```python
from build123d import *

# Parameters (mm, degrees)
SKETCH1_R           = 4
SKETCH1_R_2         = 1.5
SKETCH1_R_3         = 2.5
BOSS_EXTRUDE1_DEPTH = 4


with BuildPart() as part:
    # Sketch1 → Boss-Extrude1 (new body)
    with BuildSketch(Plane.XY):
        with BuildLine():
            Line((12.000000461, 24.00000011), (133.000000461, 24.00000011))
            ThreePointArc((133.000000461, 24.00000011), (145.000000461, 12.00000011), (133.000000461, 1.1e-07))
            Line((133.000000461, 1.1e-07), (12.000000461, 1.1e-07))
            ThreePointArc((12.000000461, 1.1e-07), (4.61e-07, 12.00000011), (12.000000461, 24.00000011))
        make_face()
        with Locations((12.000000461, 12.00000011)):
            Circle(SKETCH1_R, mode=Mode.SUBTRACT)
        with Locations((60.000000461, 5.00000011)):
            Circle(SKETCH1_R_2, mode=Mode.SUBTRACT)
        with Locations((60.000000461, 19.00000011)):
            Circle(SKETCH1_R_2, mode=Mode.SUBTRACT)
        with Locations((85.000000461, 5.00000011)):
            Circle(SKETCH1_R_2, mode=Mode.SUBTRACT)
        with Locations((85.000000461, 19.00000011)):
            Circle(SKETCH1_R_2, mode=Mode.SUBTRACT)
        with Locations((133.000000461, 12.00000011)):
            Circle(SKETCH1_R_3, mode=Mode.SUBTRACT)
        with BuildLine():
            ThreePointArc((9.729668922, 4.433322836), (12.000000461, 4.100062751), (14.270331999, 4.433322836))
            ThreePointArc((14.270331999, 4.433322836), (14.500023689, 5.017172326), (14.000000461, 5.396138381))
            ThreePointArc((14.000000461, 5.396138381), (12.000000461, 5.09992839), (10.000000461, 5.396138381))
            ThreePointArc((10.000000461, 5.396138381), (9.499977232, 5.017172326), (9.729668922, 4.433322836))
        make_face(mode=Mode.SUBTRACT)
        with BuildLine():
            ThreePointArc((19.566677735, 9.729668571), (19.899937819, 12.00000011), (19.566677735, 14.270331648))
            ThreePointArc((19.566677735, 14.270331648), (18.982828244, 14.500023338), (18.603862189, 14.00000011))
            ThreePointArc((18.603862189, 14.00000011), (18.90007218, 12.00000011), (18.603862189, 10.00000011))
            ThreePointArc((18.603862189, 10.00000011), (18.982828244, 9.499976882), (19.566677735, 9.729668571))
        make_face(mode=Mode.SUBTRACT)
        with BuildLine():
            ThreePointArc((14.270331999, 19.566677384), (12.000000461, 19.899937468), (9.729668922, 19.566677384))
            ThreePointArc((9.729668922, 19.566677384), (9.499977232, 18.982827894), (10.000000461, 18.603861839))
            ThreePointArc((10.000000461, 18.603861839), (12.000000461, 18.900071829), (14.000000461, 18.603861839))
            ThreePointArc((14.000000461, 18.603861839), (14.500023689, 18.982827894), (14.270331999, 19.566677384))
        make_face(mode=Mode.SUBTRACT)
        with BuildLine():
            ThreePointArc((4.433323186, 14.270331648), (4.100063102, 12.00000011), (4.433323186, 9.729668571))
            ThreePointArc((4.433323186, 9.729668571), (5.017172677, 9.499976882), (5.396138732, 10.00000011))
            ThreePointArc((5.396138732, 10.00000011), (5.099928741, 12.00000011), (5.396138732, 14.00000011))
            ThreePointArc((5.396138732, 14.00000011), (5.017172677, 14.500023338), (4.433323186, 14.270331648))
        make_face(mode=Mode.SUBTRACT)
    extrude(amount=BOSS_EXTRUDE1_DEPTH)


solid = part.part
```
For this review, take the finished solid that the model builds, in its own axes (mm). A direction names the side the tool comes from. Coordinates: 2 decimals unless noted, no trailing zeros. Order: outer loops, then holes, each group sorted by start corner. A loop starts at its lowest first (then second) coordinate and runs counter-clockwise, first axis right, second up. Notation, with made-up numbers: (30.25, 17) -> (45.25, 17) arc R21 cw to (45.25, 26) -> close; hole circle Ø1 at (62.5, 37). An arc over 180 degrees is marked (long way). Answer as CSV lines item,"result".
Q1. For faces 1 (the face through (19.9, 12, 2)), 2 (the face through (73, 0, 2)), list the 3-axis set-ups (+Z, -Z, +X, -X, +Y, -Y) from which the entire face can be reached by the end or side of a thin tool; tool diameter is ignored.
Model answer:
face 1,"+Z, -Z"
face 2,"+Z, -Z, +X, -X, -Y"
Q2. We need section A-A (y = 12). State the section outline as (x, z) points, plus the area to 3 significant figures.
Model answer:
outline,"(0, 0) -> (4.1, 0) -> (4.1, 4) -> (0, 4) -> close; (5.1, 0) -> (8, 0) -> (8, 4) -> (5.1, 4) -> close; (16, 0) -> (18.9, 0) -> (18.9, 4) -> (16, 4) -> close; (19.9, 0) -> (130.5, 0) -> (130.5, 4) -> (19.9, 4) -> close; (135.5, 0) -> (145, 0) -> (145, 4) -> (135.5, 4) -> close"
area,"520 mm2"
Q3. We need section C-C (x = 60). State the section outline as (y, z) points, plus the area to 3 significant figures.
Model answer:
outline,"(0, 0) -> (3.5, 0) -> (3.5, 4) -> (0, 4) -> close; (6.5, 0) -> (17.5, 0) -> (17.5, 4) -> (6.5, 4) -> close; (20.5, 0) -> (24, 0) -> (24, 4) -> (20.5, 4) -> close"
area,"72.0 mm2"
Q4. We need section B-B (z = 0.9). Count the separate pieces of the cut face and the enclosed holes in it, plus the area to 3 significant figures.
Model answer:
separate pieces,"1"
enclosed holes,"10"
area,"3,240 mm2"
Q5. Wall thickness on line 1 along Y through (x, z) = (85, 1.75); line 2 along X through (y, z) = (20.25, 1.9); line 3 along Y through (x, z) = (13, 0.8): over which ranges is each line inside the solid? List them lowest first. Write a range as [from, to].
Model answer:
line 1,"y = [0, 3.5], [6.5, 17.5], [20.5, 24]"
line 2,"x = [3.29, 59.17], [60.83, 84.17], [85.83, 141.71]"
line 3,"y = [0, 4.16], [5.17, 8.13], [15.87, 18.83], [19.84, 24]"
Q6. Draft analysis for pull direction Y (two halves, no side actions). For faces 3 (the face through (145, 12, 2)), 4 (the face through (74, 12, 0)), 5 (the face through (14.15, 15.373, 1.972)), state which applies: released by +Y, released by -Y, zero draft, split by the parting line, or undercut.
Model answer:
face 3,"split by the parting line"
face 4,"zero draft"
face 5,"undercut"
